Geometry: final body of the model. Coordinates: model frame, mm. Face numbers are marked on the shaded views. A direction names the side the tool comes from. Coordinates: 2 decimals unless noted, no trailing zeros. Order: outer loops, then holes, each group sorted by start corner. A loop starts at its lowest first (then second) coordinate and runs counter-clockwise, first axis right, second up. Notation, with made-up numbers: (-15, 81.5) -> (-5, 81.5) arc R25 ccw to (-5, 120.5) -> close; hole circle Ø10 at (-2, 15). An arc over 180 degrees is marked (long way). Use one line per item in the form item = value.
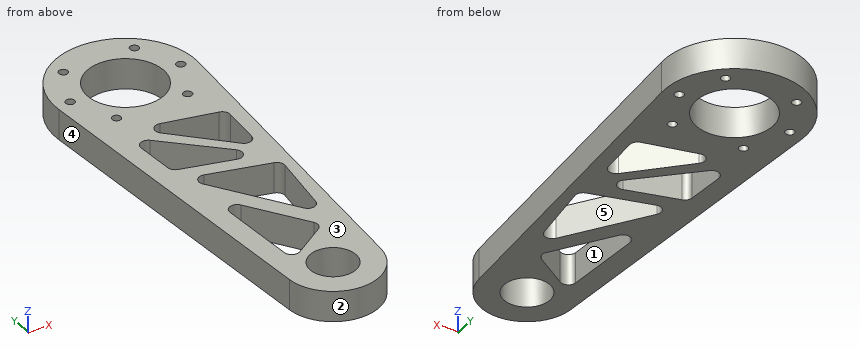
```python
from build123d import *

# Parameters (mm, degrees)
EXTRUDE_1_DEPTH     = 12
SKETCH_2_R          = 1.75
CUT_EXTRUDE_1_DEPTH = 15
SKETCH_3_R          = 15
CUT_EXTRUDE_2_DEPTH = 152.010761206
SKETCH_4_R          = 9
CUT_EXTRUDE_3_DEPTH = 152.010761206
CUT_EXTRUDE_4_DEPTH = 46
FILLET_1_R          = 3


with BuildPart() as part:
    # 草图1 → 凸台-拉伸1 (new body)
    with BuildSketch(Plane.XY):
        with BuildLine():
            Line((-17.951873532, -131.315384615), (-27.426473452, -2.009615385))
            ThreePointArc((-27.426473452, -2.009615385), (0, 27.5), (27.426473452, -2.009615385))
            Line((27.426473452, -2.009615385), (17.951873532, -131.315384615))
            ThreePointArc((17.951873532, -131.315384615), (0, -148), (-17.951873532, -131.315384615))
        make_face()
    extrude(amount=EXTRUDE_1_DEPTH)

    # 草图2 → 切除-拉伸1 (cut)
    with BuildSketch(Plane.XY.offset(12)):
        with Locations((-13.980630511, 16.661466638)):
            Circle(SKETCH_2_R)
        with Locations((-21.75, 0)):
            Circle(SKETCH_2_R)
        with Locations((-13.980630511, -16.661466638)):
            Circle(SKETCH_2_R)
        with Locations((13.980630511, -16.661466638)):
            Circle(SKETCH_2_R)
        with Locations((21.75, 0)):
            Circle(SKETCH_2_R)
        with Locations((13.980630511, 16.661466638)):
            Circle(SKETCH_2_R)
    extrude(amount=-CUT_EXTRUDE_1_DEPTH, mode=Mode.SUBTRACT)

    # 草图3 → 切除-拉伸2 (cut, through all)
    with BuildSketch(Plane.XY.offset(12)):
        Circle(SKETCH_3_R)
    extrude(amount=-CUT_EXTRUDE_2_DEPTH, mode=Mode.SUBTRACT)

    # 草图4 → 切除-拉伸3 (cut, through all)
    with BuildSketch(Plane.XY.offset(12)):
        with Locations((0, -130)):
            Circle(SKETCH_4_R)
    extrude(amount=-CUT_EXTRUDE_3_DEPTH, mode=Mode.SUBTRACT)

    # 草图5 → 切除-拉伸4 (cut)
    with BuildSketch(Plane.XY.offset(12)):
        Polygon((-13.435471405, -25.082066527), (19.516134608, -32.237272404), (17.727418447, -56.648996486), align=None)
        Polygon((-17.358092238, -28.828340185), (-15.578532958, -53.783302593), (17.727418447, -62.299703149), align=None)
        Polygon((-15.56602545, -59.74235485), (18.480575735, -68.448141084), (13.945389013, -103.211738941), align=None)
        Polygon((-13.572905823, -74.67479367), (9.289595148, -108.350537584), (-10.226621526, -121.600119355), align=None)
    extrude(amount=-CUT_EXTRUDE_4_DEPTH, mode=Mode.SUBTRACT)

    # 圆角1
    fillet_1_edges = [part.edges().sort_by_distance(p)[0] for p in [
        (13.945389013, -103.211738941, 6),
        (-15.56602545, -59.74235485, 6),
        (18.480575735, -68.448141084, 6),
        (-17.358092238, -28.828340185, 6),
        (17.727418447, -62.299703149, 6),
        (-15.578532958, -53.783302593, 6),
        (9.289595148, -108.350537584, 6),
        (-10.226621526, -121.600119355, 6),
        (-13.572905823, -74.67479367, 6),
        (17.727418447, -56.648996486, 6),
        (-13.435471405, -25.082066527, 6),
        (19.516134608, -32.237272404, 6),
    ]]
    fillet(fillet_1_edges, radius=FILLET_1_R)


solid = part.part
```
1) Section A-A, the plane y = 0. Output: boundary loops of the cut face in (x, z).
Results found:
outline = (-27.5, 0) -> (-23.5, 0) -> (-23.5, 12) -> (-27.5, 12) -> close; (-20, 0) -> (-15, 0) -> (-15, 12) -> (-20, 12) -> close; (15, 0) -> (20, 0) -> (20, 12) -> (15, 12) -> close; (23.5, 0) -> (27.5, 0) -> (27.5, 12) -> (23.5, 12) -> close
2) Section C-C, the plane x = 21.75. Output: boundary loops of the cut face in (y, z), and give its area (3 significant figures).
Results found:
outline = (-79.48, 0) -> (-1.75, 0) -> (-1.75, 12) -> (-79.48, 12) -> close; (1.75, 0) -> (16.83, 0) -> (16.83, 12) -> (1.75, 12) -> close
area = 1,110 mm2
3) Pull-direction query (Y, two-part tool) for the marked faces 3, 4 and 5; classes: released by +Y, released by -Y, zero draft, split by the parting line, or undercut.
Results found:
face_3 = zero draft
face_4 = released by -Y
face_5 = undercut
4) Contact query for flat-ended pins moving along their axis: P1, Ø5.5, axis at x = 21.75, y = 0, coming from the -Z side; P2, Ø5, axis at x = -15.5, z = 8.5, coming from the +Y side; P3, Ø5, axis at y = -60.5, z = 6.5, coming from the +X side; P4, Ø4, axis at x = -11, z = 9.5, coming from the -Y side. Output: stop coordinate, or through.
Results found:
P1 = 0
P2 = 24.23
P3 = 23.32
P4 = -145.59
5) Section D-D, the plane z = 2. Give the number of separate pieces and of enclosed holes in the cut face, and give its area (3 significant figures).
Results found:
separate_pieces = 1
enclosed_holes = 12
area = 4,820 mm2
6) Section B-B, the plane x = 4. Output: boundary loops of the cut face in (y, z), and give its area (3 significant figures).
Results found:
outline = (-147.55, 0) -> (-138.06, 0) -> (-138.06, 12) -> (-147.55, 12) -> close; (-121.94, 0) -> (-111.94, 0) -> (-111.94, 12) -> (-121.94, 12) -> close; (-100.56, 0) -> (-88.56, 0) -> (-88.56, 12) -> (-100.56, 12) -> close; (-64.75, 0) -> (-58.79, 0) -> (-58.79, 12) -> (-64.75, 12) -> close; (-49.2, 0) -> (-42.74, 0) -> (-42.74, 12) -> (-49.2, 12) -> close; (-28.87, 0) -> (-14.46, 0) -> (-14.46, 12) -> (-28.87, 12) -> close; (14.46, 0) -> (27.21, 0) -> (27.21, 12) -> (14.46, 12) -> close
area = 853 mm2
7) Material intervals for probe 1 along X at (y, z) = (-40, 4); probe 2 along X at (y, z) = (1, 9); probe 3 along X at (y, z) = (3.5, 5.25), sorted ascending. Write a range as from..to.
Results found:
probe_1 = -24.64..-16.56, -5.65..1.29, 18.95..24.64
probe_2 = -27.48..-23.19, -20.31..-14.97, 14.97..20.31, 23.19..27.48
probe_3 = -27.28..-14.59, 14.59..27.28
8) Access query for the marked faces 1 and 2. Directions: +Z, -Z, +X, -X, +Y, -Y. A direction counts if a zero-diameter tool reaches every point of the face in a straight line with its end or side. Return the directions, or none.
Results found:
face_1 = +Z, -Z
face_2 = +Z, -Z, -Y
